Job drawing, mm, ordinate dimensions from the low corner. One solid piece. A direction names the side the tool comes from. Give positions to 0.01 mm unless a question says otherwise; leave off trailing zeros. Write each loop counter-clockwise with the first axis right and the second up, starting at its lowest first coordinate (ties: lowest second). Pieces come first, ordered by that corner, then holes. Notation, with made-up numbers: (-28, 19) -> (-18, 19) arc R20 ccw to (-18, 29) -> close; hole circle Ø5 at (-31.75, 9.25). An arc over 180 degrees is marked (long way). One line per question, with ' | ' between items. Start each with the question number.
(1) Band-saw the part on A-A, the plane x = 22.5. Give the cut face in (y, z).
(2) Band-saw the part on B-B, the plane z = 23. Give the cut face in (x, y), and give its area (4 significant figures).
(3) Band-saw the part on D-D, the plane x = 30. Give the cut face in (y, z), and give its area (3 significant figures).
(4) Band-saw the part on C-C, the plane y = 15. Give the cut face in (x, z).
(5) Tool access for the marked faces 1 and 2: list every direction of +Z, -Z, +X, -X, +Y, -Y with a clear straight run to the whole face (end or side of a thin tool).
(6) Pin check, flat tips, straight feed: P1, Ø9, axis at y = 15, z = 23, coming from the -X side; P2, Ø6.5, axis at x = 22.5, y = 15, coming from the -Z side. Stop position of each tip, or through.
(7) Pull direction X, two halves, no side cores. Call the marked faces 3, 4 and 5: released by +X, released by -X, zero draft, split by the parting line, or undercut.
(8) Drill centre lines: probe 1 along X at (y, z) = (8.25, 8); probe 2 along Z at (x, y) = (30, 11.75); probe 3 along Y at (x, z) = (22.5, 1.8). Where is each one in solid material? Low to high. Write a range as from..to.
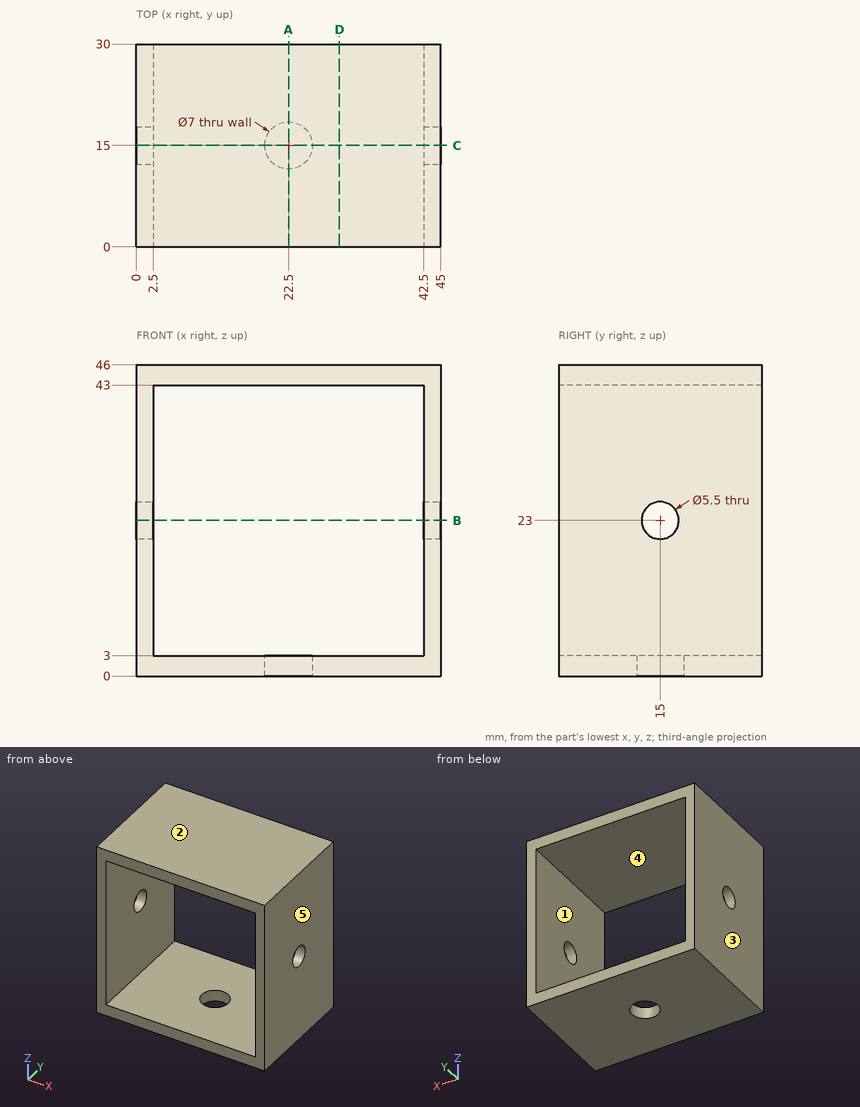
Results:
1) outline: (0, 0) -> (11.5, 0) -> (11.5, 3) -> (0, 3) -> close; (0, 43) -> (30, 43) -> (30, 46) -> (0, 46) -> close; (18.5, 0) -> (30, 0) -> (30, 3) -> (18.5, 3) -> close
2) outline: (0, 0) -> (2.5, 0) -> (2.5, 12.25) -> (0, 12.25) -> close; (0, 17.75) -> (2.5, 17.75) -> (2.5, 30) -> (0, 30) -> close; (42.5, 0) -> (45, 0) -> (45, 12.25) -> (42.5, 12.25) -> close; (42.5, 17.75) -> (45, 17.75) -> (45, 30) -> (42.5, 30) -> close | area: 122.5 mm²
3) outline: (0, 0) -> (30, 0) -> (30, 3) -> (0, 3) -> close; (0, 43) -> (30, 43) -> (30, 46) -> (0, 46) -> close | area: 180 mm²
4) outline: (0, 0) -> (19, 0) -> (19, 3) -> (2.5, 3) -> (2.5, 20.25) -> (0, 20.25) -> close; (0, 25.75) -> (2.5, 25.75) -> (2.5, 43) -> (42.5, 43) -> (42.5, 25.75) -> (45, 25.75) -> (45, 46) -> (0, 46) -> close; (26, 0) -> (45, 0) -> (45, 20.25) -> (42.5, 20.25) -> (42.5, 3) -> (26, 3) -> close
5) face 1: +Y, -Y | face 2: +Z, +X, -X, +Y, -Y
6) P1: stops at x = 0 | P2: stops at z = 43
7) face 3: released by -X | face 4: undercut | face 5: released by +X
8) probe 1: x = 0..2.5, 42.5..45 | probe 2: z = 0..3, 43..46 | probe 3: y = 0..11.5, 18.5..30
